Geometry: final body of the model. Coordinates: model frame, mm. Face numbers are marked on the shaded views. A direction names the side the tool comes from. Coordinates: 2 decimals unless noted, no trailing zeros. Write each loop counter-clockwise with the first axis right and the second up, starting at its lowest first coordinate (ties: lowest second). Pieces come first, ordered by that corner, then holes. Notation, with made-up numbers: (9, 25) - (61, 25) arc R30 ccw to (61, 58) - close; hole circle Ø11 at (-6.75, -20.5). An arc over 180 degrees is marked (long way). Answer as a JSON object with one key per item and string values. Group by question number.
Item 1: Line query: line 1 along Z through (x, y) = (85.5, 33); line 2 along Y through (x, z) = (45.5, 74.5); line 3 along Y through (x, z) = (141, 7). Output: solid intervals per line, ascending. Write a range as from..to.
Item 2: Section C-C on y = 42.5. Return loops of the section in (x, z), and give its area (3 significant figures).
Item 3: Section A-A on y = 22. Return loops of the section in (x, z), and give its area (3 significant figures).
Item 4: First-contact query: pin 1 Ø12 at (x, y) = (107.5, 25) entering from +Z; pin 2 Ø10 at (x, y) = (66, 28) entering from -Z. Flat tips, straight axial feed; report the tip coordinate or a pass-through.
Item 5: Section B-B on x = 49.45. Return loops of the section in (y, z).
Item 6: Section D-D on z = 87. Return loops of the section in (x, y), and give its area (3 significant figures).
Item 7: Set-up query: the marked faces 4 and 5. Return all of +Z, -Z, +X, -X, +Y, -Y with unobstructed straight access to the full face (end or side cutting, diameter ignored); none if empty.
Item 8: Mould query, pull axis X, two halves, no side actions, for the marked faces 1, 2 and 3. Classes: pulls with the +X half, pulls with the -X half, needs draft (parallel to the pull), parting line crosses it, or undercut.
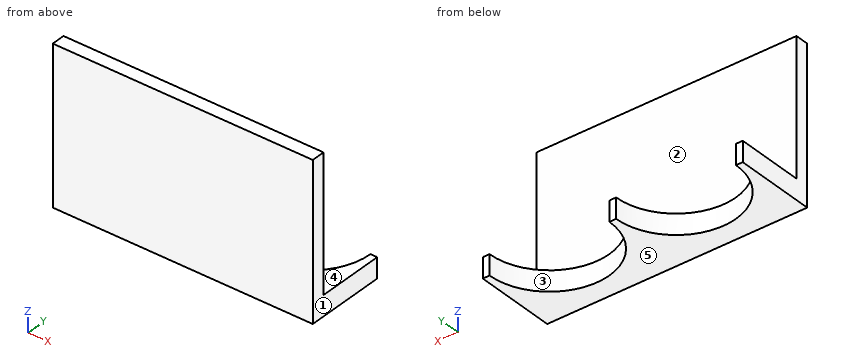
```python
from build123d import *

# Parameters (mm, degrees)
BOSS_EXTRUDE2_DEPTH = 15
SKETCH8_W           = 192.8
SKETCH8_H           = 10
BOSS_EXTRUDE3_DEPTH = 100


with BuildPart() as part:
    # Sketch7 → Boss-Extrude2 (new body)
    with BuildSketch(Plane.XY):
        with BuildLine():
            Line((0, 10), (0, 60))
            Line((0, 60), (5, 60))
            ThreePointArc((5, 60), (49.45, 15.55), (93.9, 60))
            Line((93.9, 60), (98.9, 60))
            ThreePointArc((98.9, 60), (143.35, 15.55), (187.8, 60))
            Line((187.8, 60), (192.8, 60))
            Line((192.8, 60), (192.8, 0))
            Line((192.8, 0), (0, 0))
            Line((0, 0), (0, 10))
        make_face()
    extrude(amount=BOSS_EXTRUDE2_DEPTH)

    # Sketch8 → Boss-Extrude3 (add)
    with BuildSketch(Plane.XY.offset(15)):
        with Locations((96.4, 5)):
            Rectangle(SKETCH8_W, SKETCH8_H)
    extrude(amount=BOSS_EXTRUDE3_DEPTH)


solid = part.part
```
Checks:
{
 "1": {"line 1": "0..15", "line 2": "0..10", "line 3": "0..15.61"},
 "2": {"outline": "(0, 0) - (8.59, 0) - (8.59, 15) - (0, 15) - close; (90.31, 0) - (102.49, 0) - (102.49, 15) - (90.31, 15) - close; (184.21, 0) - (192.8, 0) - (192.8, 15) - (184.21, 15) - close", "area": "440 mm^2"},
 "3": {"outline": "(0, 0) - (26.39, 0) - (26.39, 15) - (0, 15) - close; (72.51, 0) - (120.29, 0) - (120.29, 15) - (72.51, 15) - close; (166.41, 0) - (192.8, 0) - (192.8, 15) - (166.41, 15) - close", "area": "1,510 mm^2"},
 "4": {"pin 1": "z = 15", "pin 2": "through"},
 "5": {"outline": "(0, 0) - (15.55, 0) - (15.55, 15) - (10, 15) - (10, 115) - (0, 115) - close"},
 "6": {"outline": "(0, 0) - (192.8, 0) - (192.8, 10) - (0, 10) - close", "area": "1,930 mm^2"},
 "7": {"face 4": "+Z, +X, -X, +Y", "face 5": "-Z, +X, -X, +Y, -Y"},
 "8": {"face 1": "pulls with the +X half", "face 2": "needs draft", "face 3": "undercut"}
}
